Here's the drawing with two shaded views (mm, measured from the low corner). I have some questions. Round coordinates to 2 decimals unless told otherwise and drop trailing zeros. Loops run counter-clockwise (first coordinate to the right, second up) from the corner with the lowest first, then second, coordinate; pieces in that order, holes last.
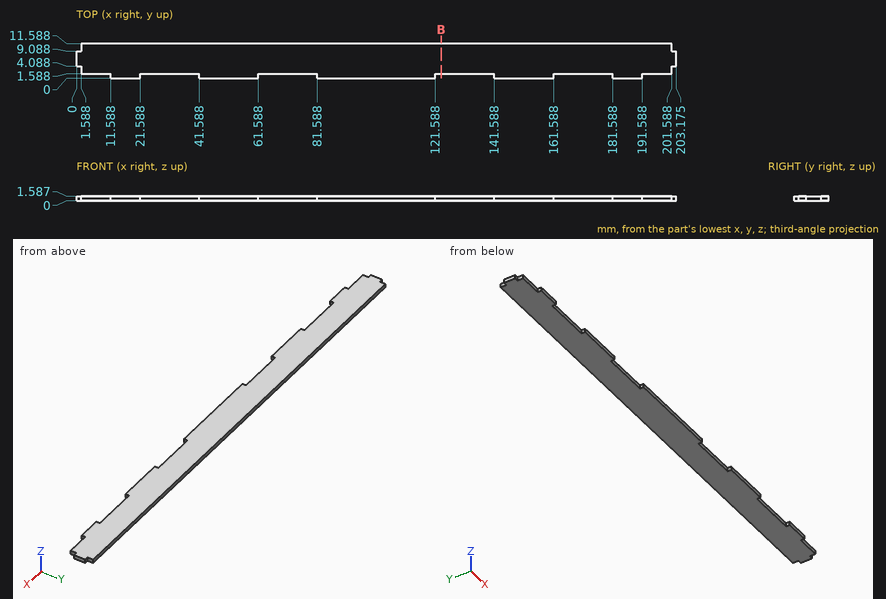
(1) Will these pins go through, and if not, where does the flat tip stop? P1, Ø0.8, axis at x = 168.5, z = 0.5, coming from the -Y side; P2, Ø0.8, axis at y = 10, z = 1, coming from the -X side; P3, Ø0.5, axis at y = 0.5, z = 0.5, coming from the +X side.
Worked answers:
P1: stops at y = 1.59
P2: stops at x = 1.59
P3: stops at x = 191.59
(2) If I drill on line 1 (X direction, y = 1.5, z = 0.4); line 2 (Y direction, x = 24, z = 0.35); line 3 (X direction, y = 10.5, z = 0.9), over which ranges is the centre line in solid material (lowest first)?
Worked answers:
line 1: x = 11.59 to 21.59, 41.59 to 61.59, 81.59 to 121.59, 141.59 to 161.59, 181.59 to 191.59
line 2: y = 1.59 to 11.59
line 3: x = 1.59 to 201.59
(3) If we section it at B-B, the plane x = 123.5: List the corners of the cut face in (y, z) for me.
Worked answers:
outline: (1.59, 0) - (11.59, 0) - (11.59, 1.59) - (1.59, 1.59) - close
